CAD build for the part. Positions are in the model's coordinates, mm. Give positions to 0.01 mm unless a question says otherwise; leave off trailing zeros. Loops run counter-clockwise (first coordinate to the right, second up) from the corner with the lowest first, then second, coordinate; pieces in that order, holes last.
```python
from build123d import *

# Parameters (mm, degrees)
SKETCH1_R           = 2.5
BOSS_EXTRUDE1_DEPTH = 10


with BuildPart() as part:
    # Sketch1 → Boss-Extrude1 (new body)
    with BuildSketch(Plane.XY):
        with BuildLine():
            Line((0, 5), (-50, 5))
            Line((-50, 5), (-57.880486008, 2.880486008))
            Line((-57.880486008, 2.880486008), (-50, -5))
            Line((-50, -5), (0, -5))
            ThreePointArc((0, -5), (5, 0), (0, 5))
        make_face()
        Circle(SKETCH1_R, mode=Mode.SUBTRACT)
    extrude(amount=BOSS_EXTRUDE1_DEPTH)


solid = part.part
```
1. Saw through at B-B, the plane z = 5. List the corners of the cut face in (x, y), and give its area (3 significant figures).
Responses:
outline: (-57.88, 2.88) - (-50, -5) - (0, -5) arc R5 ccw to (0, 5) - (-50, 5) - close; hole circle Ø5 at (0, 0)
area: 559 mm2
2. Probe line 1 along X through (y, z) = (2.25, 8.25); line 2 along X through (y, z) = (-2.25, 5.5); line 3 along X through (y, z) = (2.75, 7.5). List the from-to ranges inside material, lowest first.
Responses:
line 1: x = -57.25 to -1.09, 1.09 to 4.47
line 2: x = -52.75 to -1.09, 1.09 to 4.47
line 3: x = -57.75 to 4.18
3. Saw through at A-A, the plane y = 0. List the corners of the cut face in (x, z), and give its area (3 significant figures).
Responses:
outline: (-55, 0) - (-2.5, 0) - (-2.5, 10) - (-55, 10) - close; (2.5, 0) - (5, 0) - (5, 10) - (2.5, 10) - close
area: 550 mm2
4. Pull direction X, two halves, no side cores. Call faces 1 (the face through (-27, 0, 10)), 2 (the face through (-54, -1, 5)), 3 (the face through (-0.54, -2.44, 4.93)): released by +X, released by -X, zero draft, split by the parting line, or undercut.
Responses:
face 1: zero draft
face 2: released by -X
face 3: undercut
5. Drop flat-ended pins along their axis: pin 1 (2 mm diameter, centred on y = 3.5, z = 6, fed in from +X); pin 2 (3 mm diameter, centred on y = 0, z = 3.5, fed in from -X); pin 3 (3 mm diameter, centred on y = -2, z = 1.5, fed in from +X). Give the stop position or say it passes through.
Responses:
pin 1: stops at x = 4.33
pin 2: stops at x = -56.5
pin 3: stops at x = 4.97
6. Saw through at C-C, the plane y = -4. List the corners of the cut face in (x, z).
Responses:
outline: (-51, 0) - (3, 0) - (3, 10) - (-51, 10) - close
